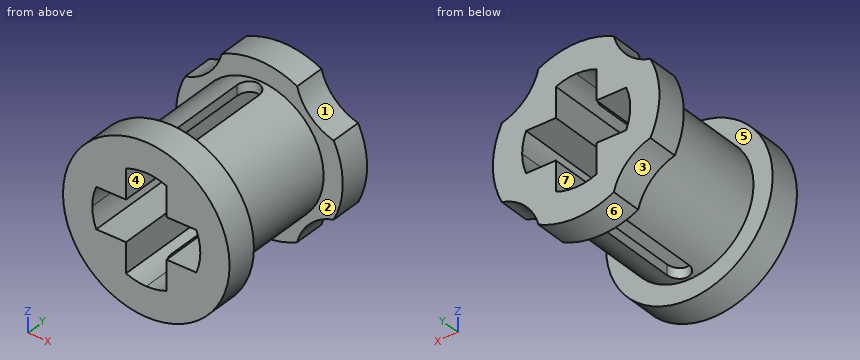
from build123d import *

# Parameters (mm, degrees)
SKETCH1_R           = 2.85
MIDDLE_BODY_DEPTH   = 2.55
SKETCH2_R           = 3.7
OUTER_RIM_DEPTH     = 1.4
AXLE_CUT_DEPTH      = 7.556104026
AXLE_CUT_DEPTH_BACK = 7.556104026
SKETCH3_W           = 1.8
SKETCH3_H           = 1.8
SLOT_CUT_DEPTH      = 7.556104026
SLOT_CUT_DEPTH_BACK = 7.556104026
SKETCH5_R           = 2.24600999
SCALLOP_CUT_DEPTH   = 1.4


with BuildPart() as part:
    # Sketch1 → Middle Body (new, symmetric)
    with BuildSketch(Plane(origin=(0, 0, 0), x_dir=(1, 0, 0), z_dir=(0, 1, 0))):
        with Locations(Location((0, 0, 0), (0, 0, 270))):
            Circle(SKETCH1_R)
    extrude(amount=MIDDLE_BODY_DEPTH, both=True)

    # Sketch2 → Outer Rim (add)
    with BuildSketch(Plane.XZ.offset(2.55)):
        with Locations(Location((0, 0, 0), (0, 0, 270))):
            Circle(SKETCH2_R)
    outer_rim = extrude(amount=OUTER_RIM_DEPTH)

    # Mirror1: Outer Rim across plane
    add(outer_rim.mirror(Plane.ZX))

    # Sketch3 → Axle Cut (cut, two sides: drawn at the far end of the back side and taken through both)
    with BuildSketch(Plane(origin=(0, 0, 0), x_dir=(1, 0, 0), z_dir=(0, 1, 0)).offset(-AXLE_CUT_DEPTH_BACK)):
        with BuildLine():
            Line((-0.9, 0.9), (0.9, 0.9))
            Line((0.9, 0.9), (0.9, 2.224859546))
            ThreePointArc((0.9, 2.224859546), (0.45844143, 2.355808026), (0, 2.4))
            ThreePointArc((0, 2.4), (-0.45844143, 2.355808026), (-0.9, 2.224859546))
            Line((-0.9, 2.224859546), (-0.9, 0.9))
        make_face()
        with BuildLine():
            Line((-2.224859546, -0.9), (-0.9, -0.9))
            Line((-0.9, -0.9), (-0.9, 0.9))
            Line((-0.9, 0.9), (-2.224859546, 0.9))
            ThreePointArc((-2.224859546, 0.9), (-2.355808026, 0.45844143), (-2.4, 0))
            ThreePointArc((-2.4, 0), (-2.355808026, -0.45844143), (-2.224859546, -0.9))
        make_face()
        Rectangle(SKETCH3_W, SKETCH3_H)
        with BuildLine():
            Line((0.9, -2.224859546), (0.9, -0.9))
            Line((0.9, -0.9), (-0.9, -0.9))
            Line((-0.9, -0.9), (-0.9, -2.224859546))
            ThreePointArc((-0.9, -2.224859546), (-0.45844143, -2.355808026), (0, -2.4))
            ThreePointArc((0, -2.4), (0.45844143, -2.355808026), (0.9, -2.224859546))
        make_face()
        with BuildLine():
            Line((0.9, -0.9), (2.224859546, -0.9))
            ThreePointArc((2.224859546, -0.9), (2.355808026, -0.45844143), (2.4, 0))
            ThreePointArc((2.4, 0), (2.355808026, 0.45844143), (2.224859546, 0.9))
            Line((2.224859546, 0.9), (0.9, 0.9))
            Line((0.9, 0.9), (0.9, -0.9))
        make_face()
    extrude(amount=AXLE_CUT_DEPTH + AXLE_CUT_DEPTH_BACK, mode=Mode.SUBTRACT)

    # Sketch4 → Slot Cut (cut, two sides: drawn at the far end of the back side and taken through both)
    with BuildSketch(Plane.XY.offset(-SLOT_CUT_DEPTH_BACK)):
        with BuildLine():
            Line((-0.5, -1.9), (-0.5, 1.9))
            ThreePointArc((-0.5, 1.9), (0, 2.4), (0.5, 1.9))
            Line((0.5, 1.9), (0.5, -1.9))
            ThreePointArc((0.5, -1.9), (0, -2.4), (-0.5, -1.9))
        make_face()
    extrude(amount=SLOT_CUT_DEPTH + SLOT_CUT_DEPTH_BACK, mode=Mode.SUBTRACT)

    # Sketch5 → Scallop Cut (cut)
    with BuildSketch(Plane(origin=(0, 3.95, 0), x_dir=(1, 0, 0), z_dir=(0, 1, 0))):
        with Locations((3.850910595, 3.850910595)):
            Circle(SKETCH5_R)
        with Locations((3.850910595, -3.850910595)):
            Circle(SKETCH5_R)
        with Locations((-3.850910595, -3.850910595)):
            Circle(SKETCH5_R)
        with Locations((-3.850910595, 3.850910595)):
            Circle(SKETCH5_R)
    extrude(amount=-SCALLOP_CUT_DEPTH, mode=Mode.SUBTRACT)


solid = part.part
Model file for the job. Use its own axes, mm. Face numbers are marked on the shaded views. A direction names the side the tool comes from. Coordinates: 2 decimals unless noted, no trailing zeros. Order: outer loops, then holes, each group sorted by start corner. A loop starts at its lowest first (then second) coordinate and runs counter-clockwise, first axis right, second up. Notation, with made-up numbers: M 53.25,-0.75 L 73.25,-0.75 A31 ccw 73.25,37.25 Z; hole C 30,-9.5 d8. An arc over 180 degrees is marked long. Return JSON: item names as keys, results as strings.
1. Saw through at A-A (y = 2.75). Give the cut face in (x, z), and give its area (3 significant figures).
Ans:
{"outline": "M -3.3,-1.67 A2.25 cw -1.67,-3.3 A3.7 ccw 1.67,-3.3 A2.25 cw 3.3,-1.67 A3.7 ccw 3.3,1.67 A2.25 cw 1.67,3.3 A3.7 ccw -1.67,3.3 A2.25 cw -3.3,1.67 A3.7 ccw Z; hole M -2.22,-0.9 L -0.9,-0.9 L -0.9,-2.22 A2.4 ccw 0.9,-2.22 L 0.9,-0.9 L 2.22,-0.9 A2.4 ccw 2.22,0.9 L 0.9,0.9 L 0.9,2.22 A2.4 ccw -0.9,2.22 L -0.9,0.9 L -2.22,0.9 A2.4 ccw Z", "area": "26.3 mm^2"}
2. Saw through at C-C (y = 1.25). Give the cut face in (x, z), and give its area (3 significant figures).
Ans:
{"outline": "M -2.22,-0.9 A2.4 cw -2.22,0.9 L -0.9,0.9 L -0.9,2.22 A2.4 cw -0.5,2.35 L -0.5,2.81 A2.85 ccw -0.5,-2.81 L -0.5,-2.35 A2.4 cw -0.9,-2.22 L -0.9,-0.9 Z; M 0.5,-2.81 A2.85 ccw 0.5,2.81 L 0.5,2.35 A2.4 cw 0.9,2.22 L 0.9,0.9 L 2.22,0.9 A2.4 cw 2.22,-0.9 L 0.9,-0.9 L 0.9,-2.22 A2.4 cw 0.5,-2.35 Z", "area": "11.0 mm^2"}
3. Tool access for the marked faces 1, 2, 3 and 4: list every direction of +Z, -Z, +X, -X, +Y, -Y with a clear straight run to the whole face (end or side of a thin tool).
Ans:
{"face 1": "+Z, +X, +Y", "face 2": "none", "face 3": "-Z, -X, +Y", "face 4": "+Y, -Y"}
4. Drill centre lines: probe 1 along Y at (x, z) = (0.5, 3.25); probe 2 along X at (y, z) = (2.25, 0.25); probe 3 along X at (y, z) = (-3.5, -0.75). Where is each one in solid material? Low to high.
Ans:
{"probe 1": "-3.95 to -2.55, 2.55 to 3.95", "probe 2": "-2.84 to -2.39, 2.39 to 2.84", "probe 3": "-3.62 to -2.28, 2.28 to 3.62"}
5. Saw through at B-B (z = -0.25). Give the cut face in (x, y).
Ans:
{"outline": "M -3.69,-3.95 L -2.39,-3.95 L -2.39,3.95 L -3.69,3.95 L -3.69,2.55 L -2.84,2.55 L -2.84,-2.55 L -3.69,-2.55 Z; M 2.39,-3.95 L 3.69,-3.95 L 3.69,-2.55 L 2.84,-2.55 L 2.84,2.55 L 3.69,2.55 L 3.69,3.95 L 2.39,3.95 Z"}
6. Flat gauge pins, fed straight in: pin 1 (1.5 mm diameter, centred on x = -2, y = -2, fed in from +Z); pin 2 (1.5 mm diameter, centred on y = 0, z = 1, fed in from +X); pin 3 (0.5 mm diameter, centred on y = 0.5, z = -2.5, fed in from +X). Where does each tip first touch, or does it go through?
Ans:
{"pin 1": "z = 3.39", "pin 2": "x = 2.84", "pin 3": "x = 1.75"}
7. Saw through at D-D (x = -0.25). Give the cut face in (y, z), and give its area (3 significant figures).
Ans:
{"outline": "M -3.95,-3.69 L -2.55,-3.69 L -2.55,-2.84 L -2.33,-2.84 L -2.33,-2.39 L -3.95,-2.39 Z; M -3.95,2.39 L -2.33,2.39 L -2.33,2.84 L -2.55,2.84 L -2.55,3.69 L -3.95,3.69 Z; M 2.33,-2.84 L 2.55,-2.84 L 2.55,-3.69 L 3.95,-3.69 L 3.95,-2.39 L 2.33,-2.39 Z; M 2.33,2.39 L 3.95,2.39 L 3.95,3.69 L 2.55,3.69 L 2.55,2.84 L 2.33,2.84 Z", "area": "7.70 mm^2"}
8. Pull direction Z, two halves, no side cores. Call the marked faces 5, 6 and 7: +Z half, -Z half, draft (parallel to the pull), parting line (faces both ways), or undercut.
Ans:
{"face 5": "draft", "face 6": "-Z half", "face 7": "undercut"}
